```python
from build123d import *

# Parameters (mm, degrees)
SKETCH_1_R          = 11
EXTRUDE_1_DEPTH     = 8
FILLET_1_R          = 100
EXTRUDE_2_DEPTH     = 10
FILLET_2_R          = 10
CHAMFER_1_SIZE      = 5
SKETCH_4_R          = 13
CUT_EXTRUDE_1_DEPTH = 3.5


with BuildPart() as part:
    # Sketch 1 → Extrude 1 (new body)
    with BuildSketch(Plane.XY):
        Polygon((0, 0), (0, 280), (861.751390409, 0), align=None)
        with Locations((200, 100)):
            Circle(SKETCH_1_R, mode=Mode.SUBTRACT)
    extrude(amount=EXTRUDE_1_DEPTH)

    # Fillet 1
    fillet_1_edges = [part.edges().sort_by_distance(p)[0] for p in [
        (861.751390409, 0, 4),
    ]]
    fillet(fillet_1_edges, radius=FILLET_1_R)

    # Sketch 2 → Extrude 2 (add)
    with BuildSketch(Plane.XY):
        with BuildLine():
            Line((0, 0), (230.376238942, 0))
            ThreePointArc((230.376238942, 0), (329.145073001, 84.356553496), (261.277938379, 195.10565163))
            Line((261.277938379, 195.10565163), (0, 280))
            Line((0, 280), (0, 0))
        make_face()
        Polygon((10, 266.236180795), (10, 35.358983849), (122.241374643, 229.766747442), align=None, mode=Mode.SUBTRACT)
        with BuildLine():
            Line((30, 10), (230.376238942, 10))
            ThreePointArc((230.376238942, 10), (319.268189595, 85.920898146), (258.187768435, 185.595086467))
            Line((258.187768435, 185.595086467), (151.410485182, 220.289128906))
            Line((151.410485182, 220.289128906), (30, 10))
        make_face(mode=Mode.SUBTRACT)
    extrude(amount=-EXTRUDE_2_DEPTH)

    # Fillet 2
    fillet_2_edges = [part.edges().sort_by_distance(p)[0] for p in [
        (30, 10, -5),
        (10, 266.236180795, -5),
        (10, 35.358983849, -5),
        (122.241374643, 229.766747442, -5),
        (151.410485182, 220.289128906, -5),
    ]]
    fillet(fillet_2_edges, radius=FILLET_2_R)

    # Chamfer 1
    chamfer_1_edges = [part.edges().sort_by_distance(p)[0] for p in [
        (130.63896919, 237.552825815, 8),
        (329.145073001, 84.356553496, 8),
        (130.63896919, 237.552825815, -10),
        (329.145073001, 84.356553496, -10),
        (115.188119471, 0, -10),
        (115.188119471, 0, 8),
    ]]
    chamfer(chamfer_1_edges, length=CHAMFER_1_SIZE)

    # Sketch 4 → Cut-Extrude 1 (cut)
    with BuildSketch(Plane(origin=(0, 0, 0), x_dir=(-1, 0, 0), z_dir=(0, 0, -1))):
        with Locations((-200, 100)):
            Circle(SKETCH_4_R)
    extrude(amount=-CUT_EXTRUDE_1_DEPTH, mode=Mode.SUBTRACT)


solid = part.part
```
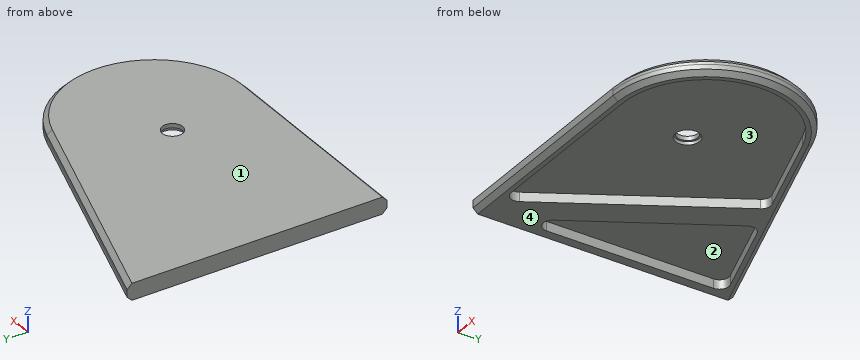
Geometry check sheet. Reference: the model listing, model coordinates, mm. Face numbers are marked on the shaded views. A direction names the side the tool comes from. Round coordinates to 2 decimals unless told otherwise and drop trailing zeros. Order: outer loops, then holes, each group sorted by start corner. A loop starts at its lowest first (then second) coordinate and runs counter-clockwise, first axis right, second up. Notation, with made-up numbers: (5, 9.25) -> (63, 9.25) arc R16 cw to (63, 15.25) -> close; hole circle Ø11 at (86, 52.5). An arc over 180 degrees is marked (long way). Return JSON: item names as keys, results as strings. Group by question number.
Q1. Gauge pin test, flat ends, axial feed: pin 1 (4 mm diameter, centred on x = 293.5, z = -6.5, fed in from -Y); pin 2 (10 mm diameter, centred on x = 292, y = 50, fed in from -Z); pin 3 (5 mm diameter, centred on x = 184, z = -6, fed in from +Y). Record the tip position at first contact, or that the pin passes through.
Q2. Section check C-C, the plane x = 165. Record the boundary of the cut face in (y, z).
Q3. Tool access check on the marked faces 1 and 2. Record the directions out of +Z, -Z, +X, -X, +Y, -Y that give a thin tool (end or side, any length) a straight path to the whole face; none if there is none.
Q4. Material ranges on probe 1 along X at (y, z) = (98.5, -2.5); probe 2 along X at (y, z) = (140, -8.75); probe 3 along Z at (x, y) = (63, 218), recorded low to high. Write a range as from..to.
Q5. Release check for a two-part mould opening along X. For the marked faces 3 and 4 record: released by +X, released by -X, zero draft, split by the parting line, or undercut.
Q6. Section check D-D, the plane y = 257.5. Record the boundary of the cut face in (x, z), plus the area to 3 significant figures.
Q7. Section check A-A, the plane y = 100. Record the boundary of the cut face in (x, z), plus the area to 3 significant figures.
Q8. Section check B-B, the plane x = 200. Record the boundary of the cut face in (y, z), plus the area to 3 significant figures.
Numbers:
{
 "1": {"pin 1": "y = 21.38", "pin 2": "z = 0", "pin 3": "y = 220.96"},
 "2": {"outline": "(0, -5) -> (5, -10) -> (10, -10) -> (10, 0) -> (215.87, 0) -> (215.87, -10) -> (221.13, -10) -> (226.39, -5) -> (226.39, 3) -> (221.13, 8) -> (5, 8) -> (0, 3) -> close"},
 "3": {"face 1": "+Z, +X, -X, +Y, -Y", "face 2": "-Z"},
 "4": {"probe 1": "0..10, 46.45..81.1, 320.36..330.36", "probe 2": "0..10, 70.41..105.06, 311..317.92", "probe 3": "0..8"},
 "5": {"face 3": "undercut", "face 4": "zero draft"},
 "6": {"outline": "(0, -10) -> (11.36, -10) -> (11.36, 0) -> (36.89, 0) -> (36.89, -10) -> (53.07, -10) -> (69.25, -5) -> (69.25, 3) -> (53.07, 8) -> (0, 8) -> close", "area": "910 mm^2"},
 "7": {"outline": "(0, -10) -> (10, -10) -> (10, 0) -> (47.32, 0) -> (47.32, -10) -> (81.96, -10) -> (81.96, 0) -> (187, 0) -> (187, 3.5) -> (189, 3.5) -> (189, 8) -> (0, 8) -> close; (211, 3.5) -> (213, 3.5) -> (213, 0) -> (320.38, 0) -> (320.38, -10) -> (325.38, -10) -> (330.38, -5) -> (330.38, 3) -> (325.38, 8) -> (211, 8) -> close", "area": "2,970 mm^2"},
 "8": {"outline": "(0, -5) -> (5, -10) -> (10, -10) -> (10, 0) -> (87, 0) -> (87, 3.5) -> (89, 3.5) -> (89, 8) -> (5, 8) -> (0, 3) -> close; (111, 3.5) -> (113, 3.5) -> (113, 0) -> (204.5, 0) -> (204.5, -10) -> (209.76, -10) -> (215.02, -5) -> (215.02, 3) -> (209.76, 8) -> (111, 8) -> close", "area": "1,680 mm^2"}
}
